```python
from build123d import *

# Parameters (mm, degrees)
CHAMFER1_SIZE  = 7
CHAMFER1_SIZE2 = 1.875644347
FILLET1_R      = 0.3


with BuildPart() as part:
    # Sketch1 → Revolve1 (revolve)
    with BuildSketch(Plane.XY, mode=Mode.PRIVATE) as revolve1_sk:
        Polygon((0, 0), (200, 0), (200, 8), (8, 8), (8, 10), (0, 10), align=None)
    revolve(revolve1_sk.sketch.rotate(Axis((0, 0, 0), (1, 0, 0)), 90), axis=Axis((0, 0, 0), (1, 0, 0)))

    # Chamfer1
    chamfer1_edges = [part.edges().sort_by_distance(p)[0] for p in [
        (200, 0, -8),
    ]]
    chamfer1_side = [part.faces().sort_by_distance(p)[0] for p in [
        (104, 0, -8),
    ]]
    chamfer(chamfer1_edges, length=CHAMFER1_SIZE, length2=CHAMFER1_SIZE2, reference=chamfer1_side[0])

    # Fillet1
    fillet1_edges = [part.edges().sort_by_distance(p)[0] for p in [
        (193, 0, -8),
        (200, 0, -6.124355653),
    ]]
    fillet(fillet1_edges, radius=FILLET1_R)


solid = part.part
```
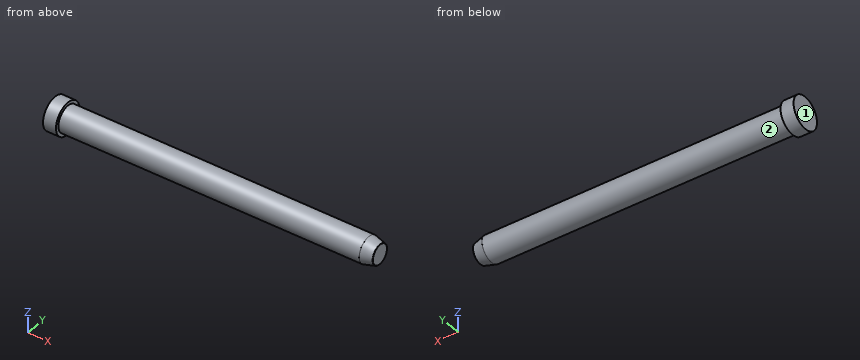
Work out the finished part from the listing and answer in its coordinate system (mm). Face numbers are marked on the shaded views. A direction names the side the tool comes from. Coordinates: 2 decimals unless noted, no trailing zeros. Loops run counter-clockwise (first coordinate to the right, second up) from the corner with the lowest first, then second, coordinate; pieces in that order, holes last.
1) Consider probe 1 along X at (y, z) = (6.5, 6); probe 2 along Z at (x, y) = (28, -1.75); probe 3 along Z at (x, y) = (83.5, -4.5). Determine where each line is inside the solid, lowest interval first.
Results:
probe 1: x = 0 to 8
probe 2: z = -7.81 to 7.81
probe 3: z = -6.61 to 6.61
2) Section A-A (x = 88.5) is taken. Give the vertices of the cut face in (y, z), plus the area to 3 significant figures.
Results:
outline: circle Ø16 at (0, 0)
area: 201 mm2
3) For the marked faces 1 and 2, determine the directions among +Z, -Z, +X, -X, +Y, -Y from which every point of the face is accessible in a straight line to the end or side of a thin tool.
Results:
face 1: +Z, -Z, -X, +Y, -Y
face 2: +X
4) Flat-ended cylindrical pins translate along their axes: pin 1 (4 mm diameter, centred on x = 169.5, y = -2.5, fed in from +Z); pin 2 (8 mm diameter, centred on x = 158.5, z = 5.5, fed in from +Y); pin 3 (3 mm diameter, centred on x = 168.5, y = -6, fed in from -Z). Find the tip coordinate at first contact, or state that the pin passes through.
Results:
pin 1: stops at z = 7.98
pin 2: stops at y = 7.86
pin 3: stops at z = -6.61
